Input: part model. Units: mm. Frame: model coordinates. A direction names the side the tool comes from. Give positions to 0.01 mm unless a question says otherwise; leave off trailing zeros. Loops run counter-clockwise (first coordinate to the right, second up) from the corner with the lowest first, then second, coordinate; pieces in that order, holes last. Notation, with made-up numbers: (63.25, 64) - (111.25, 64) arc R19 ccw to (111.25, 79) - close; hole circle Ø1 at (42.25, 53). An arc over 180 degrees is marked (long way). Answer as a JSON object with one key per item and string values.
from build123d import *

# Parameters (mm, degrees)
SKETCH1_W           = 134.7
SKETCH1_H           = 119.2
BOSS_EXTRUDE1_DEPTH = 1.2
FILLET1_R           = 10
FILLET2_R           = 4


with BuildPart() as part:
    # Sketch1 → Boss-Extrude1 (new body)
    with BuildSketch(Plane(origin=(0, 0, 0), x_dir=(1, 0, 0), z_dir=(0, 1, 0))):
        with Locations((67.35, 59.6)):
            Rectangle(SKETCH1_W, SKETCH1_H)
        Polygon((122.7, 109.2), (67.35, 61.462466726), (12, 109.2), align=None, mode=Mode.SUBTRACT)
        Polygon((10, 107.2), (10, 12), (65.190534979, 59.6), align=None, mode=Mode.SUBTRACT)
        Polygon((12, 10), (122.7, 10), (67.35, 57.737533274), align=None, mode=Mode.SUBTRACT)
        Polygon((124.7, 107.2), (124.7, 12), (69.509465021, 59.6), align=None, mode=Mode.SUBTRACT)
    extrude(amount=BOSS_EXTRUDE1_DEPTH)

    # Fillet1
    fillet1_edges = [part.edges().sort_by_distance(p)[0] for p in [
        (67.35, 0.6, -61.462466726),
        (65.190534979, 0.6, -59.6),
        (67.35, 0.6, -57.737533274),
        (69.509465021, 0.6, -59.6),
    ]]
    fillet(fillet1_edges, radius=FILLET1_R)

    # Fillet2
    fillet2_edges = [part.edges().sort_by_distance(p)[0] for p in [
        (12, 0.6, -109.2),
        (122.7, 0.6, -109.2),
        (10, 0.6, -107.2),
        (10, 0.6, -12),
        (122.7, 0.6, -10),
        (12, 0.6, -10),
        (124.7, 0.6, -107.2),
        (124.7, 0.6, -12),
    ]]
    fillet(fillet2_edges, radius=FILLET2_R)


solid = part.part
Item 1: Mould query, pull axis X, two halves, no side actions, for faces 1 (the face through (74.82, 0.61, -59.72)), 2 (the face through (66, 1.2, -60)). Classes: released by +X, released by -X, zero draft, split by the parting line, or undercut.
Geometry check:
{"face 1": "undercut", "face 2": "zero draft"}
Item 2: Cut plane A-A (y = 0.45). Return loops of the section in (x, z), then the cut area to 3 significant figures.
Geometry check:
{"outline": "(0, -119.2) - (134.7, -119.2) - (134.7, 0) - (0, 0) - close; hole (10, -98.47) arc R4 ccw to (16.61, -101.5) - (56.41, -67.17) arc R10 ccw to (56.41, -52.03) - (16.61, -17.7) arc R4 ccw to (10, -20.73) - close; hole (20.15, -102.17) arc R4 ccw to (22.76, -109.2) - (111.94, -109.2) arc R4 ccw to (114.55, -102.17) - (73.88, -67.1) arc R10 ccw to (60.82, -67.1) - close; hole (20.15, -17.03) - (60.82, -52.1) arc R10 ccw to (73.88, -52.1) - (114.55, -17.03) arc R4 ccw to (111.94, -10) - (22.76, -10) arc R4 ccw to start; hole (78.29, -67.17) - (118.09, -101.5) arc R4 ccw to (124.7, -98.47) - (124.7, -20.73) arc R4 ccw to (118.09, -17.7) - (78.29, -52.03) arc R10 ccw to start", "area": "5,770 mm2"}
Item 3: Access query for faces 3 (the face through (66, 0, -60)), 4 (the face through (94.5, 0.59, -84.88)). Directions: +Z, -Z, +X, -X, +Y, -Y. A direction counts if a zero-diameter tool reaches every point of the face in a straight line with its end or side. Return the directions, or none.
Geometry check:
{"face 3": "+Z, -Z, +X, -X, -Y", "face 4": "+Y, -Y"}
Item 4: Cut plane D-D (z = -31). Return loops of the section in (x, y), then the cut area to 3 significant figures.
Geometry check:
{"outline": "(0, 0) - (10, 0) - (10, 1.2) - (0, 1.2) - close; (32.03, 0) - (36.35, 0) - (36.35, 1.2) - (32.03, 1.2) - close; (98.35, 0) - (102.67, 0) - (102.67, 1.2) - (98.35, 1.2) - close; (124.7, 0) - (134.7, 0) - (134.7, 1.2) - (124.7, 1.2) - close", "area": "34.4 mm2"}
Item 5: Material intervals for line 1 (Z direction, x = 74, y = 0.25); line 2 (Z direction, x = 12.5, y = 0.1); line 3 (Z direction, x = 105, y = 0.9), sorted ascending. Write a range as [from, to].
Geometry check:
{"line 1": "z = [-119.2, -109.2], [-67.2, -52], [-10, 0]", "line 2": "z = [-119.2, -102.18], [-17.02, 0]", "line 3": "z = [-119.2, -109.2], [-93.93, -90.21], [-28.99, -25.27], [-10, 0]"}
Item 6: Cut plane B-B (z = -107.5). Return loops of the section in (x, y), then the cut area to 3 significant figures.
Geometry check:
{"outline": "(0, 0) - (19.49, 0) - (19.49, 1.2) - (0, 1.2) - close; (115.21, 0) - (134.7, 0) - (134.7, 1.2) - (115.21, 1.2) - close", "area": "46.8 mm2"}
Item 7: Cut plane C-C (x = 13). Return loops of the section in (y, z), then the cut area to 3 significant figures.
Geometry check:
{"outline": "(0, -119.2) - (1.2, -119.2) - (1.2, -102.34) - (0, -102.34) - close; (0, -16.86) - (1.2, -16.86) - (1.2, 0) - (0, 0) - close", "area": "40.5 mm2"}
